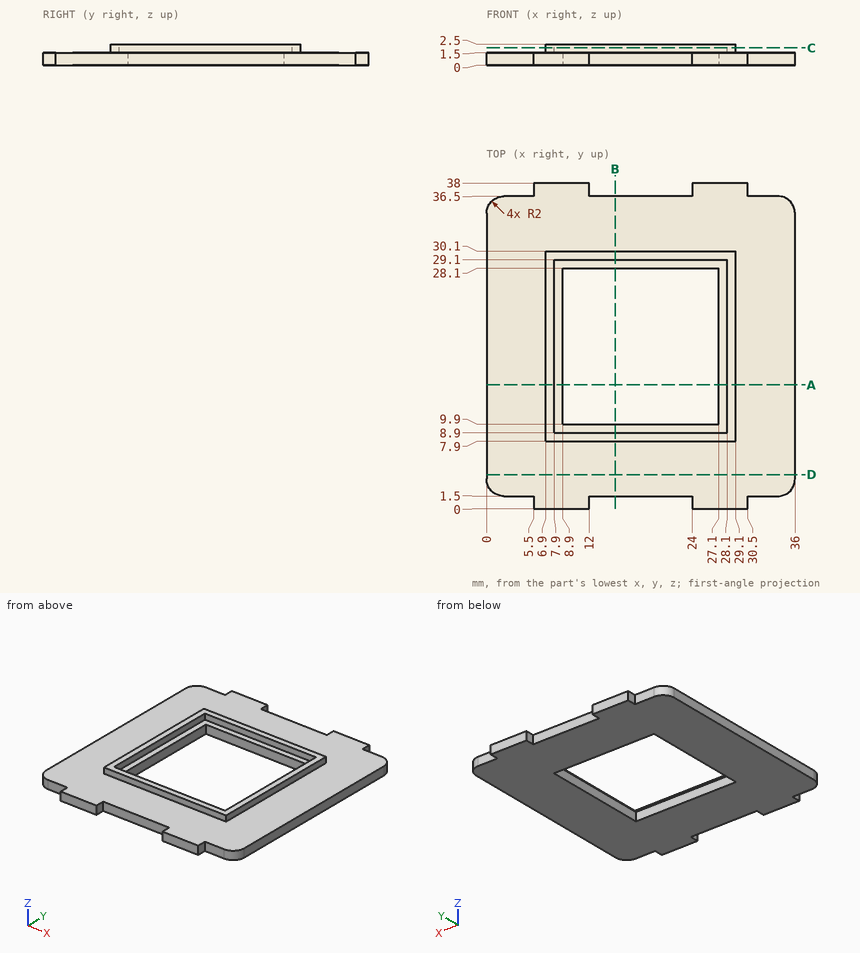
The drawing under review shows one solid part. Ordinate dimensions are in mm from its lowest x, y, z. Coordinates: 2 decimals unless noted, no trailing zeros. Order: outer loops, then holes, each group sorted by start corner. A loop starts at its lowest first (then second) coordinate and runs counter-clockwise, first axis right, second up. Notation, with made-up numbers: (70, 55) -> (118, 55) arc R7 ccw to (118, 65) -> close; hole circle Ø9 at (47, 57). An arc over 180 degrees is marked (long way). Answer as CSV lines item,"result".
Q1. We need section B-B (x = 15). State the section outline as (y, z) points, plus the area to 3 significant figures.
Model answer:
outline,"(1.5, 0) -> (9.9, 0) -> (9.9, 1.5) -> (8.9, 1.5) -> (8.9, 2.5) -> (7.9, 2.5) -> (7.9, 1.5) -> (1.5, 1.5) -> close; (28.1, 0) -> (36.5, 0) -> (36.5, 1.5) -> (30.1, 1.5) -> (30.1, 2.5) -> (29.1, 2.5) -> (29.1, 1.5) -> (28.1, 1.5) -> close"
area,"27.2 mm2"
Q2. Wall thickness on line 1 along Y through (x, z) = (9, 1.4); line 2 along Y through (x, z) = (13.5, 0.5); line 3 along X through (y, z) = (13, 0.5): over which ranges is each line inside the solid? List them lowest first. Write a range as [from, to].
Model answer:
line 1,"y = [0, 9.9], [28.1, 38]"
line 2,"y = [1.5, 9.9], [28.1, 36.5]"
line 3,"x = [0, 8.9], [27.1, 36]"
Q3. We need section A-A (y = 14.5). State the section outline as (x, z) points.
Model answer:
outline,"(0, 0) -> (8.9, 0) -> (8.9, 1.5) -> (7.9, 1.5) -> (7.9, 2.5) -> (6.9, 2.5) -> (6.9, 1.5) -> (0, 1.5) -> close; (27.1, 0) -> (36, 0) -> (36, 1.5) -> (29.1, 1.5) -> (29.1, 2.5) -> (28.1, 2.5) -> (28.1, 1.5) -> (27.1, 1.5) -> close"
Q4. We need section D-D (y = 4). State the section outline as (x, z) points.
Model answer:
outline,"(0, 0) -> (36, 0) -> (36, 1.5) -> (0, 1.5) -> close"
Q5. Clearance check with flat-ended pins moving along their axes: pin 1 Ø1.2 at (x, z) = (17, 0.5) entering from -Y; pin 2 Ø1.2 at (y, z) = (16.5, 0.5) entering from -X; pin 3 Ø1.2 at (x, z) = (16, 0.5) entering from +Y; pin 4 Ø0.5 at (x, z) = (21.5, 2) entering from -Y. State where each tip first meets the part, or that it passes through.
Model answer:
pin 1,"stops at y = 1.5"
pin 2,"stops at x = 0"
pin 3,"stops at y = 36.5"
pin 4,"stops at y = 7.9"
Q6. We need section C-C (z = 2.05). State the section outline as (x, y) points, plus the area to 3 significant figures.
Model answer:
outline,"(6.9, 7.9) -> (29.1, 7.9) -> (29.1, 30.1) -> (6.9, 30.1) -> close; hole (7.9, 8.9) -> (28.1, 8.9) -> (28.1, 29.1) -> (7.9, 29.1) -> close"
area,"84.8 mm2"
